Here's the drawing with two shaded views (mm, measured from the low corner). I have some questions. A direction names the side the tool comes from. Round coordinates to 2 decimals unless told otherwise and drop trailing zeros. Loops run counter-clockwise (first coordinate to the right, second up) from the corner with the lowest first, then second, coordinate; pieces in that order, holes last. Notation, with made-up numbers: (15, 82) -> (34, 82) arc R10 ccw to (34, 87) -> close; hole circle Ø5 at (67.5, 78). An arc over 180 degrees is marked (long way). One line per item, written item: value. Start each with the question number.
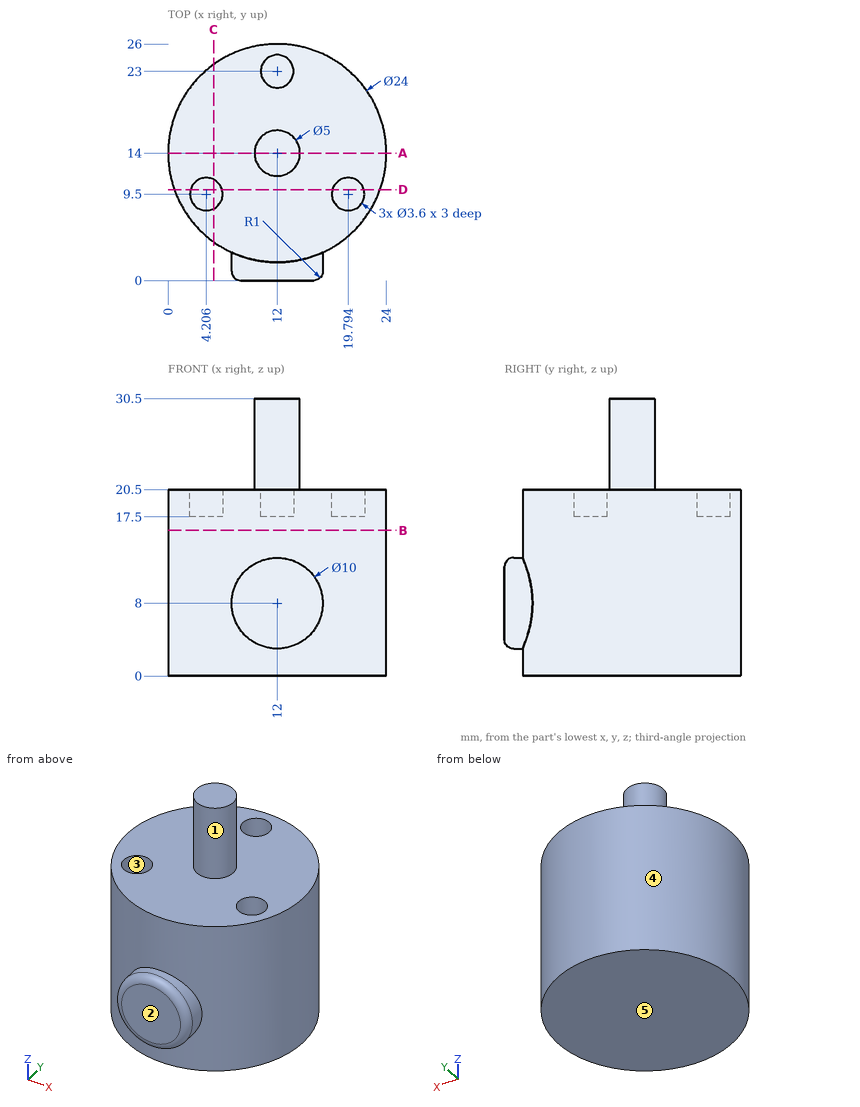
Q1. I want a section at A-A on y = 14. Please give me the cut outline in (x, z).
Q2. I want a section at D-D on y = 10. Please give me the cut outline in (x, z) (1 decimal).
Q3. I want a section at B-B on z = 16. Please give me the cut outline in (x, y).
Q4. Will these pins go through, and if not, where does the flat tip stop? P1, Ø4, axis at y = 9, z = 15.5, coming from the +X side; P2, Ø2, axis at y = 19, z = 26, coming from the +X side; P3, Ø1.5, axis at x = 3, y = 16, coming from the +Z side; P4, Ø4, axis at y = 22.5, z = 14.5, coming from the -X side.
Q5. I want a section at C-C on x = 5. Please give me the cut outline in (y, z) (1 decimal), plus the area to 3 significant figures.
Q6. Which directions (+Z, -Z, +X, -X, +Y, -Y) give clear straight access to the entire face, cutting with the end or side of a thin tool? Please do the marked faces 1 and 2.
Q7. If I drill on line 1 along Z through (x, y) = (16, 15.5); line 2 along Z through (x, y) = (5.5, 9.75); line 3 along Y through (x, z) = (12, 18.3), over which ranges is the centre line in solid material (lowest first)?
Q8. If we mould it in two halves opening along X, with no side actions, what happens to the marked faces 3, 4 and 5? For each: released by +X, released by -X, zero draft, split by the parting line, or undercut.
Answers below:
1. outline: (0, 0) -> (24, 0) -> (24, 20.5) -> (14.5, 20.5) -> (14.5, 30.5) -> (9.5, 30.5) -> (9.5, 20.5) -> (0, 20.5) -> close
2. outline: (0.7, 0) -> (23.3, 0) -> (23.3, 20.5) -> (21.5, 20.5) -> (21.5, 17.5) -> (18.1, 17.5) -> (18.1, 20.5) -> (5.9, 20.5) -> (5.9, 17.5) -> (2.5, 17.5) -> (2.5, 20.5) -> (0.7, 20.5) -> close
3. outline: circle Ø24 at (12, 14)
4. P1: stops at x = 23.62
4. P2: passes through
4. P3: stops at z = 20.5
4. P4: stops at x = 1.91
5. outline: (4.3, 0) -> (23.7, 0) -> (23.7, 20.5) -> (11.1, 20.5) -> (11.1, 17.5) -> (7.9, 17.5) -> (7.9, 20.5) -> (4.3, 20.5) -> close
5. area: 390 mm^2
6. face 1: +Z
6. face 2: +Z, -Z, +X, -X, -Y
7. line 1: z = 0 to 20.5
7. line 2: z = 0 to 17.5
7. line 3: y = 2 to 21.2, 24.8 to 26
8. face 3: undercut
8. face 4: split by the parting line
8. face 5: zero draft
